Here's how the part is built. I have some questions about the finished solid (model axes, mm). Face numbers are marked on the shaded views. A direction names the side the tool comes from. Round coordinates to 2 decimals unless told otherwise and drop trailing zeros. Write each loop counter-clockwise with the first axis right and the second up, starting at its lowest first coordinate (ties: lowest second). Pieces come first, ordered by that corner, then holes. Notation, with made-up numbers: (68.25, -6) - (90.25, -6) arc R19 ccw to (90.25, 5) - close; hole circle Ø6 at (-30, -6). An arc over 180 degrees is marked (long way). One line per item, written item: value. Start each with the question number.
Item 1: For P1, Ø9.5, axis at y = -71.5, z = -15.5, coming from the +X side; P2, Ø12, axis at y = -59, z = 8.5, coming from the -X side; P3, Ø16, axis at x = -8, y = -29, coming from the +Z side, each with a flat end and sliding along its axis, tell me the tip position at first contact or that it passes through.
Item 2: Imagine slicing it at D-D, the plane y = -24.5. Please give me the cut outline in (x, z), then the cut area to 3 significant figures.
Item 3: For the marked faces 4, 5 and 6, which set-ups out of +Z, -Z, +X, -X, +Y, -Y let a thin tool reach every point of the face, with its end or its side?
Item 4: Imagine slicing it at C-C, the plane x = -8. Please give me the cut outline in (y, z).
Item 5: Imagine slicing it at A-A, the plane x = 0. Please give me the cut outline in (y, z), then the cut area to 3 significant figures.
Item 6: Imagine slicing it at B-B, the plane z = -4.5. Please give me the cut outline in (x, y), then the cut area to 4 significant figures.
Item 7: Thinking about a two-plate mould opening in Z: for the marked faces 1, 2 and 3, which applies, released by +Z, released by -Z, zero draft, split by the parting line, or undercut?
Item 8: If I drill on line 1 (X direction, y = 3.45, z = 0); line 2 (Z direction, x = 27, y = 2.05); line 3 (Z direction, x = -14, y = 3), over which ranges is the centre line in solid material (lowest first)?
```python
from build123d import *

# Parameters (mm, degrees)
SKETCH_1_W               = 36
SKETCH_1_H               = 30
EXTRUDE_1_DEPTH          = 5
SKETCH_11_W              = 36
SKETCH_11_H              = 8
EXTRUDE_3_DEPTH          = 110
SKETCH_12_W              = 36
SKETCH_12_H              = 8
EXTRUDE_4_DEPTH          = 4
SKETCH_17_W              = 36
SKETCH_17_H              = 5
EXTRUDE_5_DEPTH          = 8
SKETCH_18_W              = 36
SKETCH_18_H              = 5
EXTRUDE_6_DEPTH          = 8
SKETCH_20_W              = 36
SKETCH_20_H              = 4
EXTRUDE_7_DEPTH          = 15
SKETCH_21_W              = 36
SKETCH_21_H              = 4
EXTRUDE_8_DEPTH          = 15
CUT_EXTRUDE_8_REACH      = 124.446
SKETCH_22_R              = 2.1
CUT_EXTRUDE_9_REACH      = 124.446
SKETCH_23_R              = 1.55
CUT_EXTRUDE_10_REACH     = 119.762
SKETCH_26_R              = 1
SKETCH_26_W              = 23.5
SKETCH_26_H              = 12
CUT_EXTRUDE_11_DEPTH     = 2
CUT_EXTRUDE_12_DEPTH     = 2
CUT_EXTRUDE_13_DEPTH     = 2
CUT_EXTRUDE_14_DEPTH     = 2
SKETCH_32_W              = 28
SKETCH_32_H              = 106
CUT_EXTRUDE_15_DEPTH     = 2
SKETCH_33_W              = 28
SKETCH_33_H              = 106
CUT_EXTRUDE_16_DEPTH     = 2
FILLET_2_R               = 1
EXTRUDE_START            = 2
SKETCH_34_W              = 32
SKETCH_34_H              = 14.000594261
SKETCH_34_R              = 1
SKETCH_34_W_2            = 23.5
SKETCH_34_H_2            = 12
EXTRUDE_12_DEPTH         = 2
CUT_EXTRUDE_START        = -2
CUT_EXTRUDE_17_OUTLINE_R = 1
CUT_EXTRUDE_17_OUTLINE_W = 23.5
CUT_EXTRUDE_17_OUTLINE_H = 12
CUT_EXTRUDE_17_DEPTH     = 2
SKETCH_36_W              = 46
SKETCH_36_H              = 5
EXTRUDE_13_DEPTH         = 15
SKETCH_37_W              = 46
SKETCH_37_H              = 5
EXTRUDE_14_DEPTH         = 15
SKETCH_38_R              = 1.55
CUT_EXTRUDE_18_DEPTH     = 5
CUT_EXTRUDE_19_REACH     = 122.437
SKETCH_39_W              = 62
SKETCH_39_H              = 10
FILLET_3_R               = 2


# Read off the part's stored shape, not the designer's step: 切除-拉伸17
with BuildPart() as part:
    # 草图1 → 凸台-拉伸1 (new body)
    with BuildSketch(Plane(origin=(0, 0, 0), x_dir=(1, 0, 0), z_dir=(0, 1, 0))):
        Rectangle(SKETCH_1_W, SKETCH_1_H)
    extrude(amount=EXTRUDE_1_DEPTH)

    # 草图11 → 凸台-拉伸3 (add)
    with BuildSketch(Plane.XZ):
        with Locations((0, 11)):
            Rectangle(SKETCH_11_W, SKETCH_11_H)
        with Locations((0, -11)):
            Rectangle(SKETCH_11_W, SKETCH_11_H)
    extrude(amount=EXTRUDE_3_DEPTH)

    # 草图12 → 凸台-拉伸4 (add)
    with BuildSketch(Plane.XZ.offset(110)):
        with Locations((0, 19)):
            Rectangle(SKETCH_12_W, SKETCH_12_H)
        with Locations((0, -19)):
            Rectangle(SKETCH_12_W, SKETCH_12_H)
    extrude(amount=-EXTRUDE_4_DEPTH)

    # 草图17 → 凸台-拉伸5 (add)
    with BuildSketch(Plane(origin=(0, 0, -15), x_dir=(-1, 0, 0), z_dir=(0, 0, -1))):
        with Locations((0, 2.5)):
            Rectangle(SKETCH_17_W, SKETCH_17_H)
    extrude(amount=EXTRUDE_5_DEPTH)

    # 草图18 → 凸台-拉伸6 (add)
    with BuildSketch(Plane.XY.offset(15)):
        with Locations((0, 2.5)):
            Rectangle(SKETCH_18_W, SKETCH_18_H)
    extrude(amount=EXTRUDE_6_DEPTH)

    # 草图20 → 凸台-拉伸7 (add)
    with BuildSketch(Plane.XY.offset(23)):
        with Locations((0, -108)):
            Rectangle(SKETCH_20_W, SKETCH_20_H)
    extrude(amount=EXTRUDE_7_DEPTH)

    # 草图21 → 凸台-拉伸8 (add)
    with BuildSketch(Plane(origin=(0, 0, -23), x_dir=(-1, 0, 0), z_dir=(0, 0, -1))):
        with Locations((0, -108)):
            Rectangle(SKETCH_21_W, SKETCH_21_H)
    extrude(amount=EXTRUDE_8_DEPTH)

    # 草图22 → 切除-拉伸8 (cut, up to next)
    with BuildSketch(Plane.XZ.offset(110), mode=Mode.PRIVATE) as cut_extrude_8_sk1:
        with Locations(Location((0, 31.819805155, 0), (0, 0, 270))):
            Circle(SKETCH_22_R)
    cut_extrude_8_tool1 = extrude(cut_extrude_8_sk1.sketch, amount=-CUT_EXTRUDE_8_REACH, mode=Mode.PRIVATE) & part.part
    # 草图22 → 切除-拉伸8 (cut, up to next)
    with BuildSketch(Plane.XZ.offset(110), mode=Mode.PRIVATE) as cut_extrude_8_sk2:
        with Locations(Location((0, -31.819805155, 0), (0, 0, 270))):
            Circle(SKETCH_22_R)
    cut_extrude_8_tool2 = extrude(cut_extrude_8_sk2.sketch, amount=-CUT_EXTRUDE_8_REACH, mode=Mode.PRIVATE) & part.part
    add(cut_extrude_8_tool1.solids().sort_by_distance((0, -110, 31.819805))[0], mode=Mode.SUBTRACT)
    add(cut_extrude_8_tool2.solids().sort_by_distance((0, -110, -31.819805))[0], mode=Mode.SUBTRACT)

    # 草图23 → 切除-拉伸9 (cut, up to next)
    with BuildSketch(Plane(origin=(0, 5, 0), x_dir=(1, 0, 0), z_dir=(0, 1, 0)), mode=Mode.PRIVATE) as cut_extrude_9_sk1:
        with Locations(Location((0, 18, 0), (0, 0, 270))):
            Circle(SKETCH_23_R)
    cut_extrude_9_tool1 = extrude(cut_extrude_9_sk1.sketch, amount=-CUT_EXTRUDE_9_REACH, mode=Mode.PRIVATE) & part.part
    # 草图23 → 切除-拉伸9 (cut, up to next)
    with BuildSketch(Plane(origin=(0, 5, 0), x_dir=(1, 0, 0), z_dir=(0, 1, 0)), mode=Mode.PRIVATE) as cut_extrude_9_sk2:
        with Locations(Location((0, -18, 0), (0, 0, 270))):
            Circle(SKETCH_23_R)
    cut_extrude_9_tool2 = extrude(cut_extrude_9_sk2.sketch, amount=-CUT_EXTRUDE_9_REACH, mode=Mode.PRIVATE) & part.part
    add(cut_extrude_9_tool1.solids().sort_by_distance((0, 5, -18))[0], mode=Mode.SUBTRACT)
    add(cut_extrude_9_tool2.solids().sort_by_distance((0, 5, 18))[0], mode=Mode.SUBTRACT)

    # 草图26 → 切除-拉伸10 (cut, up to next)
    with BuildSketch(Plane(origin=(0, 0, 0), x_dir=(-1, 0, 0), z_dir=(0, -1, 0)), mode=Mode.PRIVATE) as cut_extrude_10_sk1:
        with Locations(Location((-14, 0, 0), (0, 0, 90))):
            Circle(SKETCH_26_R)
    cut_extrude_10_tool1 = extrude(cut_extrude_10_sk1.sketch, amount=-CUT_EXTRUDE_10_REACH, mode=Mode.PRIVATE) & part.part
    # 草图26 → 切除-拉伸10 (cut, up to next)
    with BuildSketch(Plane(origin=(0, 0, 0), x_dir=(-1, 0, 0), z_dir=(0, -1, 0)), mode=Mode.PRIVATE) as cut_extrude_10_sk2:
        with Locations(Location((14, 0, 0), (0, 0, 270))):
            Circle(SKETCH_26_R)
    cut_extrude_10_tool2 = extrude(cut_extrude_10_sk2.sketch, amount=-CUT_EXTRUDE_10_REACH, mode=Mode.PRIVATE) & part.part
    # 草图26 → 切除-拉伸10 (cut, up to next)
    with BuildSketch(Plane(origin=(0, 0, 0), x_dir=(-1, 0, 0), z_dir=(0, -1, 0)), mode=Mode.PRIVATE) as cut_extrude_10_sk3:
        Rectangle(SKETCH_26_W, SKETCH_26_H)
    cut_extrude_10_tool3 = extrude(cut_extrude_10_sk3.sketch, amount=-CUT_EXTRUDE_10_REACH, mode=Mode.PRIVATE) & part.part
    add(cut_extrude_10_tool1.solids().sort_by_distance((14, 0, 0))[0], mode=Mode.SUBTRACT)
    add(cut_extrude_10_tool2.solids().sort_by_distance((-14, 0, 0))[0], mode=Mode.SUBTRACT)
    add(cut_extrude_10_tool3.solids().sort_by_distance((0, 0, 0))[0], mode=Mode.SUBTRACT)

    # 草图28 → 切除-拉伸11 (cut)
    with BuildSketch(Plane(origin=(18, 0, 0), x_dir=(0, 0, -1), z_dir=(1, 0, 0))):
        Polygon((23, 5), (-23, 5), (-23, 0), (-15, 0), (-15, -106), (-38, -106), (-38, -110), (-7, -110), (-7, 0), (7, 0), (7, -110), (38, -110), (38, -106), (15, -106), (15, 0), (23, 0), align=None)
    extrude(amount=-CUT_EXTRUDE_11_DEPTH, mode=Mode.SUBTRACT)

    # 草图29 → 切除-拉伸12 (cut)
    with BuildSketch(Plane.ZY.offset(18)):
        Polygon((23, 5), (-23, 5), (-23, 0), (-15, 0), (-15, -106), (-38, -106), (-38, -110), (-7, -110), (-7, 0), (7, 0), (7, -110), (38, -110), (38, -106), (15, -106), (15, 0), (23, 0), align=None)
    extrude(amount=-CUT_EXTRUDE_12_DEPTH, mode=Mode.SUBTRACT)

    # 草图30 → 切除-拉伸13 (cut)
    with BuildSketch(Plane(origin=(16, 0, 0), x_dir=(0, 0, -1), z_dir=(1, 0, 0))):
        Polygon((-15, 0), (-7, 0), (-7, -110), (-38, -110), (-38, -106), (-15, -106), align=None)
        Polygon((7, 0), (15, 0), (15, -106), (38, -106), (38, -110), (7, -110), align=None)
    extrude(amount=-CUT_EXTRUDE_13_DEPTH, mode=Mode.SUBTRACT)

    # 草图31 → 切除-拉伸14 (cut)
    with BuildSketch(Plane.ZY.offset(16)):
        Polygon((-7, 0), (-7, -110), (-38, -110), (-38, -106), (-15, -106), (-15, 0), align=None)
        Polygon((15, 0), (15, -106), (38, -106), (38, -110), (7, -110), (7, 0), align=None)
    extrude(amount=-CUT_EXTRUDE_14_DEPTH, mode=Mode.SUBTRACT)

    # 草图32 → 切除-拉伸15 (cut)
    with BuildSketch(Plane.XY.offset(15)):
        with Locations((0, -53)):
            Rectangle(SKETCH_32_W, SKETCH_32_H)
    extrude(amount=-CUT_EXTRUDE_15_DEPTH, mode=Mode.SUBTRACT)

    # 草图33 → 切除-拉伸16 (cut)
    with BuildSketch(Plane(origin=(0, 0, -15), x_dir=(-1, 0, 0), z_dir=(0, 0, -1))):
        with Locations((0, -53)):
            Rectangle(SKETCH_33_W, SKETCH_33_H)
    extrude(amount=-CUT_EXTRUDE_16_DEPTH, mode=Mode.SUBTRACT)

    # 圆角2
    fillet_2_edges = [part.edges().sort_by_distance(p)[0] for p in [
        (0, -110, -7),
        (0, -110, 7),
        (0, -106, 13),
        (0, -106, -13),
    ]]
    fillet(fillet_2_edges, radius=FILLET_2_R)

    # 草图34 → 凸台-拉伸12 (add)
    with BuildSketch(Plane.XZ.offset(EXTRUDE_START)):
        with Locations((0, 0.000297131)):
            Rectangle(SKETCH_34_W, SKETCH_34_H)
        with Locations(Location((14, 0, 0), (0, 0, 270))):
            Circle(SKETCH_34_R, mode=Mode.SUBTRACT)
        with Locations(Location((-14, 0, 0), (0, 0, 270))):
            Circle(SKETCH_34_R, mode=Mode.SUBTRACT)
        Rectangle(SKETCH_34_W_2, SKETCH_34_H_2, mode=Mode.SUBTRACT)
    extrude(amount=-EXTRUDE_12_DEPTH)

    # 切除-拉伸17 outline → 切除-拉伸17 (cut)
    with BuildSketch(Plane.XZ.offset(2).offset(CUT_EXTRUDE_START)):
        Polygon((-16, -7), (16, -7), (16, 7.000594261), (14, 7.000594261), (14, 7), (-14, 7), (-14, 7.000594261), (-16, 7.000594261), align=None)
        with Locations((-14, 0)):
            Circle(CUT_EXTRUDE_17_OUTLINE_R, mode=Mode.SUBTRACT)
        Rectangle(CUT_EXTRUDE_17_OUTLINE_W, CUT_EXTRUDE_17_OUTLINE_H, mode=Mode.SUBTRACT)
        with Locations((14, 0)):
            Circle(CUT_EXTRUDE_17_OUTLINE_R, mode=Mode.SUBTRACT)
    extrude(amount=CUT_EXTRUDE_17_DEPTH, mode=Mode.SUBTRACT)

    # 草图36 → 凸台-拉伸13 (add)
    with BuildSketch(Plane.ZY.offset(16)):
        with Locations((0, 2.5)):
            Rectangle(SKETCH_36_W, SKETCH_36_H)
    extrude(amount=EXTRUDE_13_DEPTH)

    # 草图37 → 凸台-拉伸14 (add)
    with BuildSketch(Plane(origin=(16, 0, 0), x_dir=(0, 0, -1), z_dir=(1, 0, 0))):
        with Locations((0, 2.5)):
            Rectangle(SKETCH_37_W, SKETCH_37_H)
    extrude(amount=EXTRUDE_14_DEPTH)

    # 草图38 → 切除-拉伸18 (cut)
    with BuildSketch(Plane.XZ):
        with Locations(Location((-27, 0, 0), (0, 0, 270))):
            Circle(SKETCH_38_R)
        with Locations(Location((27, 0, 0), (0, 0, 90))):
            Circle(SKETCH_38_R)
    extrude(amount=-CUT_EXTRUDE_18_DEPTH, mode=Mode.SUBTRACT)

    # 草图39 → 切除-拉伸19 (cut, up to next)
    with BuildSketch(Plane.XZ, mode=Mode.PRIVATE) as cut_extrude_19_sk1:
        with Locations((0, 18)):
            Rectangle(SKETCH_39_W, SKETCH_39_H)
    cut_extrude_19_tool1 = extrude(cut_extrude_19_sk1.sketch, amount=-CUT_EXTRUDE_19_REACH, mode=Mode.PRIVATE) & part.part
    # 草图39 → 切除-拉伸19 (cut, up to next)
    with BuildSketch(Plane.XZ, mode=Mode.PRIVATE) as cut_extrude_19_sk2:
        with Locations((0, -18)):
            Rectangle(SKETCH_39_W, SKETCH_39_H)
    cut_extrude_19_tool2 = extrude(cut_extrude_19_sk2.sketch, amount=-CUT_EXTRUDE_19_REACH, mode=Mode.PRIVATE) & part.part
    add(cut_extrude_19_tool1.solids().sort_by_distance((0, 0, 18))[0], mode=Mode.SUBTRACT)
    add(cut_extrude_19_tool2.solids().sort_by_distance((0, 0, -18))[0], mode=Mode.SUBTRACT)

    # 圆角3
    fillet_3_edges = [part.edges().sort_by_distance(p)[0] for p in [
        (-14, 0, -10),
        (-14, 0, 10),
        (14, 0, -10),
        (14, 0, 10),
    ]]
    fillet(fillet_3_edges, radius=FILLET_3_R)


solid = part.part
```
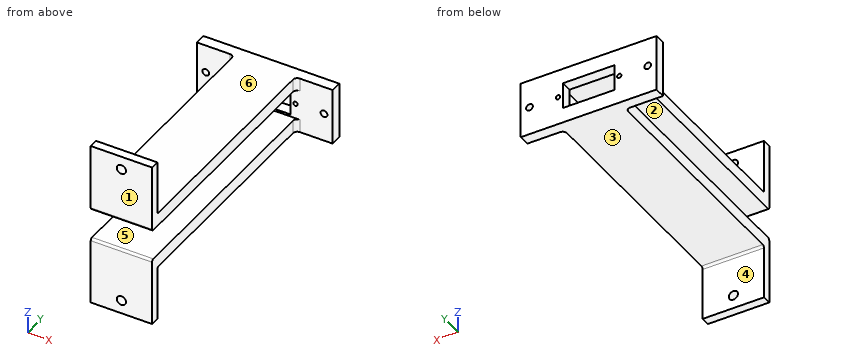
Values follow:
1. P1: stops at x = 14
1. P2: stops at x = -14
1. P3: stops at z = 13
2. outline: (-14, -13) - (14, -13) - (14, -7) - (-14, -7) - close; (-14, 7) - (14, 7) - (14, 13) - (-14, 13) - close
2. area: 336 mm^2
3. face 4: -Z, +X, -X, +Y
3. face 5: +X, -X, -Y
3. face 6: +Z, +X, -X, +Y
4. outline: (-110, -38) - (-106, -38) - (-106, -14) arc R1 cw to (-105, -13) - (5, -13) - (5, -6) - (0, -6) - (0, -7) - (-109, -7) arc R1 ccw to (-110, -8) - close; (-110, 8) arc R1 ccw to (-109, 7) - (0, 7) - (0, 6) - (5, 6) - (5, 13) - (-105, 13) arc R1 cw to (-106, 14) - (-106, 38) - (-110, 38) - close
5. outline: (-110, -38) - (-106, -38) - (-106, -33.92) - (-110, -33.92) - close; (-110, -29.72) - (-106, -29.72) - (-106, -14) arc R1 cw to (-105, -13) - (5, -13) - (5, -6) - (0, -6) - (0, -7) - (-109, -7) arc R1 ccw to (-110, -8) - close; (-110, 8) arc R1 ccw to (-109, 7) - (0, 7) - (0, 6) - (5, 6) - (5, 13) - (-105, 13) arc R1 cw to (-106, 14) - (-106, 29.72) - (-110, 29.72) - close; (-110, 33.92) - (-106, 33.92) - (-106, 38) - (-110, 38) - close
5. area: 1,560 mm^2
6. outline: (-31, 0) - (-11.75, 0) - (-11.75, 5) - (-31, 5) - close; (11.75, 0) - (31, 0) - (31, 5) - (11.75, 5) - close
6. area: 192.5 mm^2
7. face 1: zero draft
7. face 2: undercut
7. face 3: released by -Z
8. line 1: x = -31 to -28.55, -25.45 to -15, -13 to -11.75, 11.75 to 13, 15 to 25.45, 28.55 to 31
8. line 2: z = -13 to -1.55, 1.55 to 13
8. line 3: z = -13 to -1, 1 to 13
